```python
from build123d import *

# Parameters (mm, degrees)
BOSS_EXTRUDE1_DEPTH = 20
SKETCH4_W           = 5
SKETCH4_H           = 90
BOSS_EXTRUDE4_DEPTH = 5


with BuildPart() as part:
    # Sketch1 → Boss-Extrude1 (new body)
    with BuildSketch(Plane.XY):
        with BuildLine():
            Line((-80, 74.379500648), (-80, -15.620499352))
            Line((-80, -15.620499352), (-60, -15.620499352))
            ThreePointArc((-60, -15.620499352), (0, 62), (60, -15.620499352))
            Line((60, -15.620499352), (80, -15.620499352))
            Line((80, -15.620499352), (80, 74.379500648))
            Line((80, 74.379500648), (-80, 74.379500648))
        make_face()
    extrude(amount=BOSS_EXTRUDE1_DEPTH)

    # Sketch4 → Boss-Extrude4 (add)
    with BuildSketch(Plane(origin=(0, 0, 0), x_dir=(-1, 0, 0), z_dir=(0, 0, -1))):
        with Locations((77.5, 29.379500648)):
            Rectangle(SKETCH4_W, SKETCH4_H)
    extrude(amount=BOSS_EXTRUDE4_DEPTH)


solid = part.part
```
Build history of the part. All positions in model axes, mm. A direction names the side the tool comes from. Coordinates: 2 decimals unless noted, no trailing zeros. Order: outer loops, then holes, each group sorted by start corner. A loop starts at its lowest first (then second) coordinate and runs counter-clockwise, first axis right, second up.
Item 1: Saw through at A-A on y = 0. List the corners of the cut face in (x, z).
Filled in:
outline: (-80, -5) - (-75, -5) - (-75, 0) - (-62, 0) - (-62, 20) - (-80, 20) - close; (62, 0) - (80, 0) - (80, 20) - (62, 20) - close
Item 2: Saw through at C-C on z = -2.75. List the corners of the cut face in (x, y), then the cut area to 3 significant figures.
Filled in:
outline: (-80, -15.62) - (-75, -15.62) - (-75, 74.38) - (-80, 74.38) - close
area: 450 mm2
Item 3: Mould opens along Y. For faces 3 (the flat face through (-77, 30, -5)), 4 (the cylindrical face through (-1.58, 61.98, 9.86)), 5 (the flat face through (-70, -15.62, 10)) say: released by +Y, released by -Y, zero draft, split by the parting line, or undercut.
Filled in:
face 3: zero draft
face 4: undercut
face 5: released by -Y
Item 4: Drop flat-ended pins along their axis: pin 1 Ø1.5 at (y, z) = (8.5, -2) entering from +X; pin 2 Ø1.5 at (x, z) = (22, 12.5) entering from -Y; pin 3 Ø10 at (x, z) = (-12, 6.5) entering from -Y. Give the stop position or say it passes through.
Filled in:
pin 1: stops at x = -75
pin 2: stops at y = 57.68
pin 3: stops at y = 59.62
Item 5: Saw through at B-B on y = 68.5. List the corners of the cut face in (x, z).
Filled in:
outline: (-80, -5) - (-75, -5) - (-75, 0) - (80, 0) - (80, 20) - (-80, 20) - close
Item 6: Saw through at D-D on x = 0. List the corners of the cut face in (y, z), then the cut area to 3 significant figures.
Filled in:
outline: (62, 0) - (74.38, 0) - (74.38, 20) - (62, 20) - close
area: 248 mm2
Item 7: Drill centre lines: L1, parallel to X at y = 0, z = 5.25; L2, parallel to X at y = 44, z = -0.5; L3, parallel to Y at x = -0.5, z = 0.5. Where is each one in solid material? Low to high.
Filled in:
L1: x = -80 to -62, 62 to 80
L2: x = -80 to -75
L3: y = 62 to 74.38
Item 8: Tool access for faces 1 (the flat face through (70, -15.62, 10)), 2 (the flat face through (19, 60, 0)): list every direction of +Z, -Z, +X, -X, +Y, -Y with a clear straight run to the whole face (end or side of a thin tool).
Filled in:
face 1: +Z, -Z, +X, -X, -Y
face 2: -Z, +X, +Y, -Y
